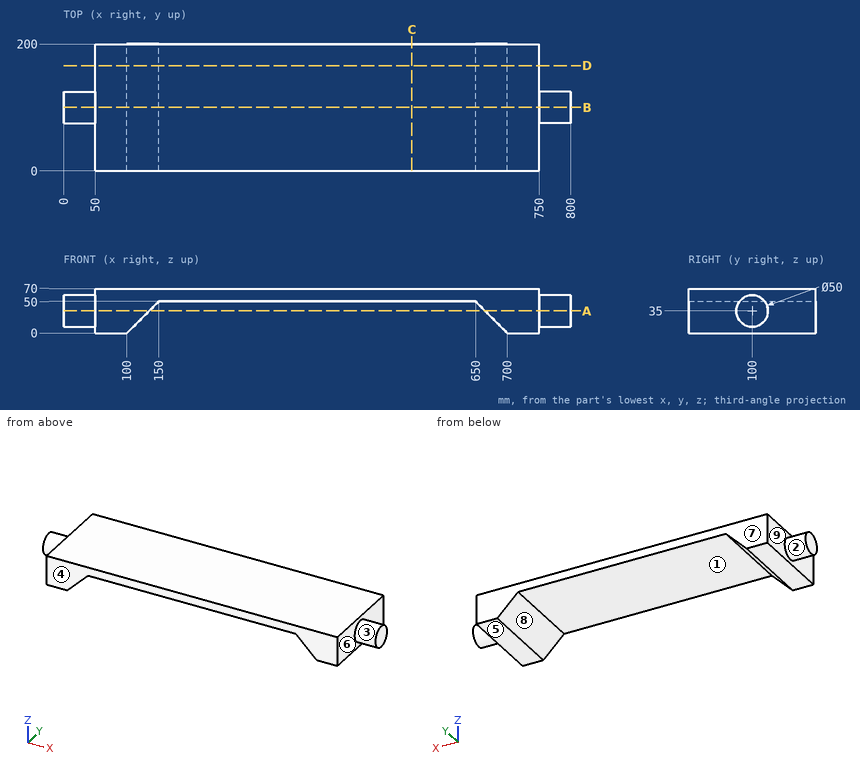
Answer from the drawing. Dimensions are ordinates in mm from the lowest x, y and z of the part. A direction names the side the tool comes from. Coordinates: 2 decimals unless noted, no trailing zeros. Loops run counter-clockwise (first coordinate to the right, second up) from the corner with the lowest first, then second, coordinate; pieces in that order, holes last. Notation, with made-up numbers: (76, -18) - (100, -18) arc R29 ccw to (100, 13) - close; hole circle Ø5 at (20, 33). An arc over 180 degrees is marked (long way). Use a Markdown table: item, result.
Item 1: Consider probe 1 along Z at (x, y) = (314.5, 111); probe 2 along X at (y, z) = (152, 24.5); probe 3 along X at (y, z) = (61, 35). Determine where each line is inside the solid, lowest interval first. Write a range as from..to.
Evaluation:
| item | result |
|---|---|
| probe 1 | z = 50..70 |
| probe 2 | x = 50..124.5, 675.5..750 |
| probe 3 | x = 50..135, 665..750 |
Item 2: For the marked faces 1, 2, 3, 4 and 5, determine the directions among +Z, -Z, +X, -X, +Y, -Y from which every point of the face is accessible in a straight line to the end or side of a thin tool.
Evaluation:
| item | result |
|---|---|
| face 1 | -Z, +Y, -Y |
| face 2 | -X |
| face 3 | +X |
| face 4 | +Z, -Z, +X, -X, -Y |
| face 5 | -Z, +X, -X, +Y, -Y |
Item 3: Find section D-D, the plane y = 166. Determine the outline of the cut face in (x, z).
Evaluation:
| item | result |
|---|---|
| outline | (50, 0) - (100, 0) - (150, 50) - (650, 50) - (700, 0) - (750, 0) - (750, 70) - (50, 70) - close |
Item 4: Given pin 1 Ø12 at (y, z) = (53.5, 36.5) entering from -X, flat-ended and moving along its own axis, determine where the tip first touches the part or whether it passes through.
Evaluation:
| item | result |
|---|---|
| pin 1 | stops at x = 50 |
Item 5: Find section C-C, the plane x = 549.5. Determine the outline of the cut face in (y, z), and give its area (3 significant figures).
Evaluation:
| item | result |
|---|---|
| outline | (0, 50) - (200, 50) - (200, 70) - (0, 70) - close |
| area | 4,000 mm2 |
Item 6: Find section B-B, the plane y = 100. Determine the outline of the cut face in (x, z).
Evaluation:
| item | result |
|---|---|
| outline | (0, 10) - (50, 10) - (50, 0) - (100, 0) - (150, 50) - (650, 50) - (700, 0) - (750, 0) - (750, 10) - (800, 10) - (800, 60) - (750, 60) - (750, 70) - (50, 70) - (50, 60) - (0, 60) - close |
Item 7: Find section A-A, the plane z = 35. Determine the outline of the cut face in (x, y), and give its area (3 significant figures).
Evaluation:
| item | result |
|---|---|
| outline | (0, 75) - (50, 75) - (50, 0) - (135, 0) - (135, 200) - (50, 200) - (50, 125) - (0, 125) - close; (665, 0) - (750, 0) - (750, 75) - (800, 75) - (800, 125) - (750, 125) - (750, 200) - (665, 200) - close |
| area | 39,000 mm2 |
Item 8: The mould has two halves that part along X. Classify the marked faces 6, 7, 8 and 9: +X half, -X half, draft (parallel to the pull), parting line (faces both ways), or undercut.
Evaluation:
| item | result |
|---|---|
| face 6 | +X half |
| face 7 | draft |
| face 8 | undercut |
| face 9 | -X half |
